The model under review builds one solid part; all positions refer to its coordinate system, in mm. Face numbers are marked on the shaded views. Round coordinates to 2 decimals unless told otherwise and drop trailing zeros. Write each loop counter-clockwise with the first axis right and the second up, starting at its lowest first coordinate (ties: lowest second). Pieces come first, ordered by that corner, then holes. Notation, with made-up numbers: (64.25, 24.25) -> (86.25, 24.25) arc R33 ccw to (86.25, 57.25) -> close; hole circle Ø1 at (-22, 52.25). An arc over 180 degrees is marked (long way). Use CSV: the item, a comma, the result in double quotes. Start each with the question number.
1) Mouldability with a two-part tool opening along Y and no side actions: class the marked faces 1 and 2 as released by +Y, released by -Y, zero draft, split by the parting line, or undercut.
2) Take a section at A-A, the plane z = 2.9. Give the boundary of the cut face in (x, y).
3) For pin 1 Ø11 at (x, y) = (22.94, 1.7) entering from -Z; pin 2 Ø4 at (x, y) = (-22.5, 5.5) entering from +Z; pin 3 Ø1.1 at (y, z) = (-2, 1.5) entering from +X; pin 4 Ø2 at (y, z) = (11, 3.5) entering from +X, all flat-tipped, find the tip position at first contact; note any pin that passes through.
4) Take a section at B-B, the plane y = 0. Give the boundary of the cut face in (x, z), then the cut area to 3 significant figures.
5) Wall thickness on probe 1 along X at (y, z) = (5.5, 1.7); probe 2 along Y at (x, z) = (-9.5, 3.15); probe 3 along Y at (x, z) = (-5, 2.6): over which ranges is each line inside the solid? List them lowest first. Write a range as [from, to].
6) Take a section at C-C, the plane x = 11. State how many separate pieces and enclosed holes the cut face has, then the cut area to 3 significant figures.
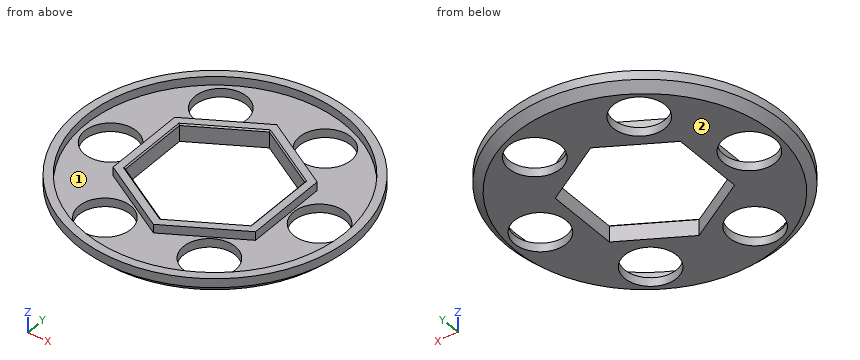
from build123d import *

# Parameters (mm, degrees)
SKETCH_R        = 31.9
SKETCH_R_2      = 6
PAD_DEPTH       = 2
SKETCH001_R     = 31.9
SKETCH001_R_2   = 30
PAD001_DEPTH    = 2
PAD002_DEPTH    = 2
CHAMFER_SIZE    = 1.9
CHAMFER001_SIZE = 0.3


with BuildPart() as part:
    # Sketch → Pad (new body)
    with BuildSketch(Plane.XY):
        Circle(SKETCH_R)
        with Locations((9.999037, 20.71278)):
            Circle(SKETCH_R_2, mode=Mode.SUBTRACT)
        with Locations((22.937312, 1.69697)):
            Circle(SKETCH_R_2, mode=Mode.SUBTRACT)
        with Locations((12.938275, -19.01581)):
            Circle(SKETCH_R_2, mode=Mode.SUBTRACT)
        with Locations((-9.999037, -20.71278)):
            Circle(SKETCH_R_2, mode=Mode.SUBTRACT)
        with Locations((-22.937312, -1.69697)):
            Circle(SKETCH_R_2, mode=Mode.SUBTRACT)
        with Locations((-12.938275, 19.01581)):
            Circle(SKETCH_R_2, mode=Mode.SUBTRACT)
        Polygon((0, 16.743158), (-14.5, 8.371579), (-14.5, -8.371579), (0, -16.743158), (14.5, -8.371579), (14.5, 8.371579), align=None, mode=Mode.SUBTRACT)
    extrude(amount=PAD_DEPTH)

    # Sketch001 (on Face15 of Pad) → Pad001 (join)
    with BuildSketch(Plane.XY.offset(2)):
        Circle(SKETCH001_R)
        Circle(SKETCH001_R_2, mode=Mode.SUBTRACT)
    extrude(amount=PAD001_DEPTH)

    # Sketch002 (on Face17 of Pad001) → Pad002 (join)
    with BuildSketch(Plane.XY.offset(2)):
        Polygon((0, 19.052559), (-16.5, 9.526279), (-16.5, -9.526279), (0, -19.052559), (16.5, -9.526279), (16.5, 9.526279), align=None)
        Polygon((0, 16.743158), (-14.5, 8.371579), (-14.5, -8.371579), (0, -16.743158), (14.5, -8.371579), (14.5, 8.371579), align=None, mode=Mode.SUBTRACT)
    extrude(amount=PAD002_DEPTH)

    # Chamfer
    chamfer_edges = [part.edges().sort_by_distance(p)[0] for p in [
        (-31.9, 0, 0),
    ]]
    chamfer(chamfer_edges, length=CHAMFER_SIZE)

    # Chamfer001
    chamfer001_edges = [part.edges().sort_by_distance(p)[0] for p in [
        (-7.25, -12.557368, 4),
        (-14.5, 0, 4),
        (-7.25, 12.557368, 4),
        (7.25, 12.557368, 4),
        (14.5, 0, 4),
        (7.25, -12.557368, 4),
    ]]
    chamfer(chamfer001_edges, length=CHAMFER001_SIZE)


solid = part.part
Values found:
1,face 1,"undercut"
1,face 2,"zero draft"
2,outline,"circle Ø63.8 at (0, 0); (-16.5, -9.53) -> (0, -19.05) -> (16.5, -9.53) -> (16.5, 9.53) -> (0, 19.05) -> (-16.5, 9.53) -> close; hole circle Ø60 at (0, 0); hole (-14.5, -8.37) -> (0, -16.74) -> (14.5, -8.37) -> (14.5, 8.37) -> (0, 16.74) -> (-14.5, 8.37) -> close"
3,pin 1,"through"
3,pin 2,"z = 2"
3,pin 3,"x = 31.86"
3,pin 4,"x = 30.29"
4,outline,"(-31.9, 1.9) -> (-30, 0) -> (-28.69, 0) -> (-28.69, 2) -> (-30, 2) -> (-30, 4) -> (-31.9, 4) -> close; (-17.18, 0) -> (-14.5, 0) -> (-14.5, 3.7) -> (-14.8, 4) -> (-16.5, 4) -> (-16.5, 2) -> (-17.18, 2) -> close; (14.5, 0) -> (17.18, 0) -> (17.18, 2) -> (16.5, 2) -> (16.5, 4) -> (14.8, 4) -> (14.5, 3.7) -> close; (28.69, 0) -> (30, 0) -> (31.9, 1.9) -> (31.9, 4) -> (30, 4) -> (30, 2) -> (28.69, 2) -> close"
4,area,"35.5 mm²"
5,probe 1,"[-31.22, -14.5], [14.5, 18.3], [27.58, 31.22]"
5,probe 2,"[-30.45, -28.46], [-13.57, -11.26], [11.26, 13.57], [28.46, 30.45]"
5,probe 3,"[-31.51, -29.58], [-16.17, -13.86], [13.86, 16.17], [29.58, 31.51]"
6,separate pieces,"4"
6,enclosed holes,"0"
6,area,"45.2 mm²"
